Could you check a few things on this model? Use its own coordinates, in mm. A direction names the side the tool comes from. Round coordinates to 2 decimals unless told otherwise and drop trailing zeros. Loops run counter-clockwise (first coordinate to the right, second up) from the corner with the lowest first, then second, coordinate; pieces in that order, holes last. Notation, with made-up numbers: (-19, 11) - (4, 11) arc R31 ccw to (4, 37) - close; hole circle Ø8 at (-0.5, 31.5). An arc over 180 degrees is marked (long way). Use one line per item in the form item = value.
```python
from build123d import *

# Parameters (mm, degrees)
SKETCH1_W           = 39.624
SKETCH1_H           = 25.4
SKETCH1_R           = 0.95
BOSS_EXTRUDE1_DEPTH = 4
SKETCH3_W           = 31.75
SKETCH3_H           = 25.4
SKETCH3_R           = 1.75
BOSS_EXTRUDE2_DEPTH = 4
SKETCH5_W           = 21.59
SKETCH5_H           = 36.5125
CUT_EXTRUDE2_DEPTH  = 44.129170453
CHAMFER1_SIZE       = 4.064
FILLET2_R           = 3.175


with BuildPart() as part:
    # Sketch1 → Boss-Extrude1 (new body)
    with BuildSketch(Plane(origin=(0, 0, 0), x_dir=(1, 0, 0), z_dir=(0, 1, 0))):
        Rectangle(SKETCH1_W, SKETCH1_H)
        with Locations(Location((-17.145, 10.16, 0), (0, 0, 270))):
            Circle(SKETCH1_R, mode=Mode.SUBTRACT)
        with Locations(Location((-17.145, -10.16, 0), (0, 0, 270))):
            Circle(SKETCH1_R, mode=Mode.SUBTRACT)
        with Locations(Location((17.145, -10.16, 0), (0, 0, 270))):
            Circle(SKETCH1_R, mode=Mode.SUBTRACT)
        with Locations(Location((17.145, 10.16, 0), (0, 0, 270))):
            Circle(SKETCH1_R, mode=Mode.SUBTRACT)
    extrude(amount=BOSS_EXTRUDE1_DEPTH)

    # Sketch3 → Boss-Extrude2 (add)
    with BuildSketch(Plane.XZ):
        with Locations((0, -25.4)):
            Rectangle(SKETCH3_W, SKETCH3_H)
        with Locations(Location((-10.795, -33.3375, 0), (0, 0, 270))):
            Circle(SKETCH3_R, mode=Mode.SUBTRACT)
        with Locations(Location((10.795, -33.3375, 0), (0, 0, 270))):
            Circle(SKETCH3_R, mode=Mode.SUBTRACT)
    extrude(amount=-BOSS_EXTRUDE2_DEPTH)

    # Sketch5 → Cut-Extrude2 (cut, through all)
    with BuildSketch(Plane.XZ):
        with Locations((0, -8.73125)):
            Rectangle(SKETCH5_W, SKETCH5_H)
    extrude(amount=-CUT_EXTRUDE2_DEPTH, mode=Mode.SUBTRACT)

    # Chamfer1
    # the kernel refuses this chamfer: 4.064 mm, written as the material it adds along each edge
    with BuildSketch(Plane(origin=(15.875, 0, -12.7), x_dir=(0.9996219169112968, 0, 0.027495876610586435), z_dir=(0, 1, 0))) as chamfer1_piece_1_section:
        Polygon((CHAMFER1_SIZE * 0.999621916911, CHAMFER1_SIZE * 0.0274958766106), (-CHAMFER1_SIZE * 0.0274958766106, CHAMFER1_SIZE * 0.999621916911), (0, 0), align=None)
    chamfer1_piece_1 = extrude(amount=4, mode=Mode.PRIVATE)
    chamfer1_piece_1 = split(chamfer1_piece_1, bisect_by=Plane(origin=(19.812, 2, -14.047586344), z_dir=(-1, 0, 0)), keep=Keep.TOP, mode=Mode.PRIVATE)
    add(chamfer1_piece_1)
    with BuildSketch(Plane(origin=(-15.875, 0, -12.7), x_dir=(-0.9996219169112968, 0, 0.027495876610586455), z_dir=(0, 1, 0))) as chamfer1_piece_2_section:
        Polygon((CHAMFER1_SIZE * 0.999621916911, -CHAMFER1_SIZE * 0.0274958766106), (-CHAMFER1_SIZE * 0.0274958766106, -CHAMFER1_SIZE * 0.999621916911), (0, 0), align=None)
    chamfer1_piece_2 = extrude(amount=4, mode=Mode.PRIVATE)
    chamfer1_piece_2 = split(chamfer1_piece_2, bisect_by=Plane(origin=(-19.812, 2, -14.047586344), z_dir=(1, 0, 0)), keep=Keep.TOP, mode=Mode.PRIVATE)
    add(chamfer1_piece_2)

    # Fillet2
    fillet2_edges = [part.edges().sort_by_distance(p)[0] for p in [
        (15.875, 2, -38.1),
        (-15.875, 2, -38.1),
        (10.795, 2, 9.525),
        (10.795, 2, -26.9875),
        (-10.795, 2, -26.9875),
        (-10.795, 2, 9.525),
        (15.875, 2, -16.764),
        (-15.875, 2, -16.764),
        (19.812, 2, -12.827),
        (-19.812, 2, -12.827),
        (19.812, 2, 12.7),
        (-19.812, 2, 12.7),
    ]]
    fillet(fillet2_edges, radius=FILLET2_R)


solid = part.part
```
1. We'd pull the mould along X, two halves only. Please class faces 4 (the face through (19.812, 2, -1)), 5 (the face through (-15.875, 2, -27)), 6 (the face through (10.795, 2, -9)), 7 (the face through (-14, 0, -12)): +X half, -X half, draft (parallel to the pull), parting line (faces both ways), or undercut.
Solution:
face_4 = +X half
face_5 = -X half
face_6 = undercut
face_7 = draft
2. Please list where these lines run through material, in increasing order: line 1 along X through (y, z) = (3.25, -10) (3 decimals); line 2 along Z through (x, y) = (-2, 1.55) (1 decimal); line 3 along X through (y, z) = (1.1, -2.5) (3 decimals).
Solution:
line_1 = -19.812 to -18.081, -16.209 to -10.795, 10.795 to 16.209, 18.081 to 19.812
line_2 = -38.1 to -27, 9.5 to 12.7
line_3 = -19.812 to -10.795, 10.795 to 19.812
3. If we section it at A-A, the plane z = -7: Write out the boundary of the cut face in (x, y) (3 decimals), plus the area to 3 significant figures.
Solution:
outline = (-19.812, 0) - (-10.795, 0) - (-10.795, 4) - (-19.812, 4) - close; (10.795, 0) - (19.812, 0) - (19.812, 4) - (10.795, 4) - close
area = 72.1 mm^2
4. If we section it at D-D, the plane y = 1.5: Count the separate pieces of the cut face and the enclosed holes in it, plus the area to 3 significant figures.
Solution:
separate_pieces = 1
enclosed_holes = 7
area = 1,010 mm^2
5. If we section it at C-C, the plane z = 10.16: Write out the boundary of the cut face in (x, y) (3 decimals), plus the area to 3 significant figures.
Solution:
outline = (-19.748, 0) - (-18.095, 0) - (-18.095, 4) - (-19.748, 4) - close; (-16.195, 0) - (16.195, 0) - (16.195, 4) - (-16.195, 4) - close; (18.095, 0) - (19.748, 0) - (19.748, 4) - (18.095, 4) - close
area = 143 mm^2
6. If we section it at B-B, the plane x = -1.5: Write out the boundary of the cut face in (y, z) (1 decimal), plus the area to 4 significant figures.
Solution:
outline = (0, -38.1) - (4, -38.1) - (4, -27) - (0, -27) - close; (0, 9.5) - (4, 9.5) - (4, 12.7) - (0, 12.7) - close
area = 57.15 mm^2
7. On a 3-axis mill with a long thin cutter (end or side, diameter ignored), from which of +Z, -Z, +X, -X, +Y, -Y can I reach the whole of each face in a straight line? I mean faces 1 (the face through (9.84, 2.03, -26.08)), 2 (the face through (-14, 4, -12)), 3 (the face through (15.875, 2, -27)). Say none if no direction works.
Solution:
face_1 = +Y, -Y
face_2 = +Z, -Z, +X, -X, +Y
face_3 = -Z, +X, +Y, -Y
8. For P1, Ø1.2, axis at y = 1, z = -28, coming from the -X side (3 decimals); P2, Ø3, axis at x = -17.145, z = -10.16, coming from the +Y side, each with a flat end and sliding along its axis, tell me the tip position at first contact or that it passes through.
Solution:
P1 = -15.875
P2 = 4
